Here's how the part is built. I have some questions about the finished solid (model axes, mm). Coordinates: 2 decimals unless noted, no trailing zeros. Write each loop counter-clockwise with the first axis right and the second up, starting at its lowest first coordinate (ties: lowest second). Pieces come first, ordered by that corner, then holes.
Item 1: I want a section at C-C (x = 7.62). Please give me the cut outline in (y, z), and give its area (3 significant figures).
Item 2: Please list where these lines run through material, in increasing order: line 1 (Z direction, x = 8.25, y = 5.5); line 2 (X direction, y = 7.75, z = -1).
Item 3: I'm going to push a flat-ended pin straight in: P1, Ø1, axis at x = 7.5, y = 7, coming from the -Z side. Where does the tip first touch, or does it pass through?
Item 4: I want a section at D-D (y = 6.75). Please give me the cut outline in (x, z), and give its area (3 significant figures).
Item 5: I want a section at B-B (y = 0). Please give me the cut outline in (x, z).
Item 6: I want a section at A-A (z = -1.25). Please give me the cut outline in (x, y), and give its area (3 significant figures).
from build123d import *

# Parameters (mm, degrees)
SKETCH001_R  = 0.35
PAD001_DEPTH = 3.5
SKETCH_W     = 10.16
SKETCH_H     = 10.16
PAD_DEPTH    = 7.62
FILLET_R     = 0.7


with BuildPart() as pad001:
    # Sketch001 → Pad001 (new body)
    with BuildSketch(Plane.XY.offset(0.5)):
        Circle(SKETCH001_R)
        with Locations((7.62, 7.62)):
            Circle(SKETCH001_R)
    extrude(amount=-PAD001_DEPTH)


with BuildPart() as obj1:
    # Sketch → Pad (new body)
    with BuildSketch(Plane.XY.offset(0.1)):
        with Locations((3.81, 3.81)):
            Rectangle(SKETCH_W, SKETCH_H)
    extrude(amount=PAD_DEPTH)

    # Fillet
    fillet_edges = [obj1.edges().sort_by_distance(p)[0] for p in [
        (8.89, -1.27, 3.91),
        (8.89, 8.89, 3.91),
        (-1.27, -1.27, 3.91),
        (-1.27, 8.89, 3.91),
    ]]
    fillet(fillet_edges, radius=FILLET_R)

    # obj1: union Pad001
    add(pad001.part)


solid = obj1.part
Answer:
1. outline: (-1.27, 0.1) - (7.27, 0.1) - (7.27, -3) - (7.97, -3) - (7.97, 0.1) - (8.89, 0.1) - (8.89, 7.72) - (-1.27, 7.72) - close
1. area: 79.6 mm2
2. line 1: z = 0.1 to 7.72
2. line 2: x = 7.3 to 7.94
3. P1: stops at z = -3
4. outline: (-1.27, 0.1) - (8.89, 0.1) - (8.89, 7.72) - (-1.27, 7.72) - close
4. area: 77.4 mm2
5. outline: (-1.27, 0.1) - (-0.35, 0.1) - (-0.35, -3) - (0.35, -3) - (0.35, 0.1) - (8.89, 0.1) - (8.89, 7.72) - (-1.27, 7.72) - close
6. outline: circle Ø0.7 at (0, 0); circle Ø0.7 at (7.62, 7.62)
6. area: 0.770 mm2
